Source: CAD feature listing. Evaluate the final solid. Frame: model axes, mm. A direction names the side the tool comes from. Give positions to 0.01 mm unless a question says otherwise; leave off trailing zeros. Order: outer loops, then holes, each group sorted by start corner. A loop starts at its lowest first (then second) coordinate and runs counter-clockwise, first axis right, second up.
1) Section B-B, the plane x = 23.5. Return loops of the section in (y, z), plus the area to 3 significant figures.
2) Section C-C, the plane y = 0. Return loops of the section in (x, z).
3) Section A-A, the plane y = 83.5. Return loops of the section in (x, z), plus the area to 3 significant figures.
4) Draft query along Y for faces 1 (the face through (45, 83, 0)), 2 (the face through (-20, 320, 0)), 3 (the face through (-1, -106, 0)), 4 (the face through (-23.304, 104.944, -35.633)). Return one class per face: released by +Y, released by -Y, zero draft, split by the parting line, or undercut.
5) Access query for faces 5 (the face through (74.927, -3.298, 0.364)), 6 (the face through (115, 320, 20)), 7 (the face through (45, -83, 0)), 8 (the face through (-85.31, -65.41, 35.37)). Directions: +Z, -Z, +X, -X, +Y, -Y. A direction counts if a zero-diameter tool reaches every point of the face in a straight line with its end or side. Return the directions, or none.
6) First-contact query: P1, Ø10, axis at y = 321, z = -3, coming from the -X side; P2, Ø10, axis at x = 48, y = 324, coming from the -Z side; P3, Ø10, axis at y = -21, z = -31, coming from the -X side. Flat tips, straight axial feed; report the tip coordinate or a pass-through.
7) Material intervals for line 1 (Z direction, x = 41, y = 74.5); line 2 (Z direction, x = 67, y = -83); line 3 (Y direction, x = 32, z = 16), sorted ascending.
8) Section D-D, the plane z = 0. Return loops of the section in (x, y).
```python
from build123d import *

# Parameters (mm, degrees)
SKETCH_1_R        = 75
EXTRUDE_296_DEPTH = 26
SKETCH_2_R        = 15
EXTRUDE_341_DEPTH = 330
SKETCH_3_W        = 267
SKETCH_3_H        = 40
EXTRUDE_488_DEPTH = 20
SKETCH_4_W        = 90
SKETCH_4_H        = 40
EXTRUDE_594_DEPTH = 106
SKETCH_5_R        = 107.5
EXTRUDE_1_DEPTH   = 19
EXTRUDE_START     = 19
SKETCH_6_R        = 107.5
EXTRUDE_2_DEPTH   = 19


with BuildPart() as part:
    # Sketch 1 → Extrude 296 (new, symmetric)
    with BuildSketch(Plane.XY):
        with Locations(Location((0, 0, 0), (0, 0, 180))):
            Circle(SKETCH_1_R)
    extrude(amount=EXTRUDE_296_DEPTH, both=True)

    # Sketch 2 → Extrude 341 (add)
    with BuildSketch(Plane(origin=(0, 0, 0), x_dir=(1, 0, 0), z_dir=(0, 1, 0))):
        with Locations(Location((0, 0, 0), (0, 0, 90))):
            Circle(SKETCH_2_R)
    extrude(amount=EXTRUDE_341_DEPTH)

    # Sketch 3 → Extrude 488 (add)
    with BuildSketch(Plane(origin=(0, 330, 0), x_dir=(-1, 0, 0), z_dir=(0, 1, 0))):
        with Locations((-113.5, 0)):
            Rectangle(SKETCH_3_W, SKETCH_3_H)
    extrude(amount=-EXTRUDE_488_DEPTH)

    # Sketch 4 → Extrude 594 (add, symmetric)
    with BuildSketch(Plane(origin=(0, 0, 0), x_dir=(1, 0, 0), z_dir=(0, 1, 0))):
        Rectangle(SKETCH_4_W, SKETCH_4_H)
    extrude(amount=EXTRUDE_594_DEPTH, both=True)

    # Sketch 5 → Extrude 1 (add)
    with BuildSketch(Plane.XY.offset(26)):
        Circle(SKETCH_5_R)
    extrude(amount=EXTRUDE_1_DEPTH)

    # Sketch 6 → Extrude 2 (add)
    with BuildSketch(Plane(origin=(0, 0, -26), x_dir=(-1, 0, 0), z_dir=(0, 0, -1)).offset(EXTRUDE_START)):
        with Locations(Location((0, 0, 0), (0, 0, 180))):
            Circle(SKETCH_6_R)
    extrude(amount=-EXTRUDE_2_DEPTH)


solid = part.part
```
From the geometry:
1. outline: (-106, -20) - (-71.22, -20) - (-71.22, -26) - (-104.9, -26) - (-104.9, -45) - (104.9, -45) - (104.9, -26) - (71.22, -26) - (71.22, -20) - (106, -20) - (106, 20) - (71.22, 20) - (71.22, 26) - (104.9, 26) - (104.9, 45) - (-104.9, 45) - (-104.9, 26) - (-71.22, 26) - (-71.22, 20) - (-106, 20) - close; (310, -20) - (330, -20) - (330, 20) - (310, 20) - close
1. area: 19,000 mm2
2. outline: (-107.5, -45) - (107.5, -45) - (107.5, -26) - (75, -26) - (75, 26) - (107.5, 26) - (107.5, 45) - (-107.5, 45) - (-107.5, 26) - (-75, 26) - (-75, -26) - (-107.5, -26) - close
3. outline: (-67.71, -45) - (67.71, -45) - (67.71, -26) - (-67.71, -26) - close; (-67.71, 26) - (67.71, 26) - (67.71, 45) - (-67.71, 45) - close; (-45, -20) - (45, -20) - (45, 20) - (-45, 20) - close
3. area: 8,750 mm2
4. face 1: undercut
4. face 2: zero draft
4. face 3: released by -Y
4. face 4: split by the parting line
5. face 5: none
5. face 6: +Z, +X, -X, +Y
5. face 7: +X, -Y
5. face 8: +Z
6. P1: stops at x = -20
6. P2: stops at z = -20
6. P3: stops at x = -106.3
7. line 1: z = -45 to -26, -20 to 20, 26 to 45
7. line 2: z = -45 to -26, 26 to 45
7. line 3: y = -106 to 106, 310 to 330
8. outline: (-45, -106) - (45, -106) - (45, -60) arc R75 ccw to (45, 60) - (45, 106) - (15, 106) - (15, 310) - (247, 310) - (247, 330) - (-20, 330) - (-20, 310) - (-15, 310) - (-15, 106) - (-45, 106) - (-45, 60) arc R75 ccw to (-45, -60) - close
